```python
from build123d import *

# Parameters (mm, degrees)
SKETCH1_R           = 11.000000098
SKETCH1_R_2         = 4.1984422
SKETCH1_R_3         = 1.56235781
BOSS_EXTRUDE1_DEPTH = 2.794
SKETCH4_R           = 5.08
BOSS_EXTRUDE2_DEPTH = 5.08
BOSS_EXTRUDE4_DEPTH = 25.4


with BuildPart() as part:
    # Sketch1 → Boss-Extrude1 (new body)
    with BuildSketch(Plane.XY):
        with Locations((-211.672901702, 6.35719782)):
            Circle(SKETCH1_R)
        with Locations((-211.672901702, 6.35719782)):
            Circle(SKETCH1_R_2, mode=Mode.SUBTRACT)
        with Locations((-211.672901702, 14.35819782)):
            Circle(SKETCH1_R_3, mode=Mode.SUBTRACT)
        with Locations((-219.673901702, 6.35719782)):
            Circle(SKETCH1_R_3, mode=Mode.SUBTRACT)
        with Locations((-211.672901702, -1.64380218)):
            Circle(SKETCH1_R_3, mode=Mode.SUBTRACT)
        with Locations((-203.671901702, 6.35719782)):
            Circle(SKETCH1_R_3, mode=Mode.SUBTRACT)
    extrude(amount=BOSS_EXTRUDE1_DEPTH)

    # Sketch4 → Boss-Extrude2 (add)
    with BuildSketch(Plane.XY.offset(2.794)):
        with Locations((-211.672901702, 6.35719782)):
            Circle(SKETCH4_R)
    extrude(amount=BOSS_EXTRUDE2_DEPTH)

    # Sketch6 → Boss-Extrude4 (add)
    with BuildSketch(Plane.XY.offset(7.874)):
        Polygon((-217.614895912, 10.703116021), (-210.880223241, 13.676074856), (-204.938229031, 9.330156654), (-205.730907491, 2.011279618), (-212.465580162, -0.961679217), (-218.407574373, 3.384238985), align=None)
    extrude(amount=BOSS_EXTRUDE4_DEPTH)


solid = part.part
```
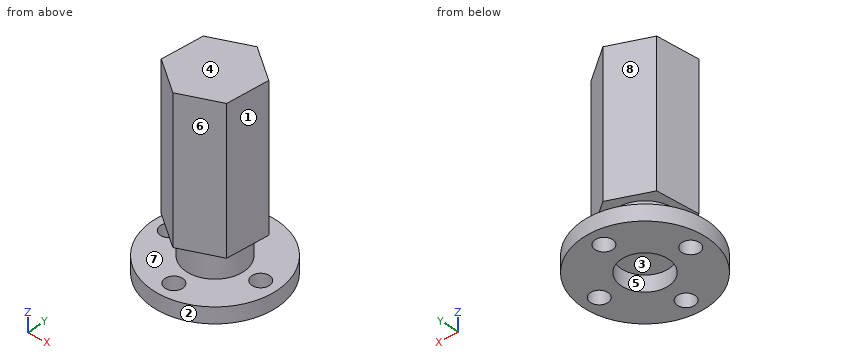
Build history of the part. All positions in model axes, mm. Face numbers are marked on the shaded views. A direction names the side the tool comes from. Give positions to 0.01 mm unless a question says otherwise; leave off trailing zeros. Order: outer loops, then holes, each group sorted by start corner. A loop starts at its lowest first (then second) coordinate and runs counter-clockwise, first axis right, second up. Notation, with made-up numbers: M 82,-9.5 L 117,-9.5 A23 cw 117,22.5 Z; hole C 45,81 d9. An arc over 180 degrees is marked long. Return JSON: item names as keys, results as strings.
Q1. Band-saw the part on D-D (z = 25). Give the cut face in (x, y), then the cut area to 3 significant figures.
Answer list:
{"outline": "M -218.41,3.38 L -212.47,-0.96 L -205.73,2.01 L -204.94,9.33 L -210.88,13.68 L -217.61,10.7 Z", "area": "141 mm^2"}
Q2. Two-plate mould, pull along X, no slides. Class the marked faces 1, 2, 3 and 4: pulls with the +X half, pulls with the -X half, needs draft (parallel to the pull), parting line crosses it, or undercut.
Answer list:
{"face 1": "pulls with the +X half", "face 2": "parting line crosses it", "face 3": "undercut", "face 4": "needs draft"}
Q3. Flat gauge pins, fed straight in: pin 1 (10 mm diameter, centred on y = -2, z = 25.5, fed in from +X); pin 2 (3 mm diameter, centred on x = -219.67, y = 6.36, fed in from +Z); pin 3 (4 mm diameter, centred on x = -211.67, y = -1.64, fed in from -Z); pin 4 (5 mm diameter, centred on x = -213, z = 18, fed in from -Y). Where does each tip first touch, or does it go through?
Answer list:
{"pin 1": "stops at x = -205.62", "pin 2": "passes through", "pin 3": "stops at z = 0", "pin 4": "stops at y = -0.96"}
Q4. 3-axis set-ups, long thin cutter, end or side, ignore diameter. For the marked faces 5, 6, 7 and 8: which of +Z, -Z, +X, -X, +Y, -Y reach the whole face in a straight line?
Answer list:
{"face 5": "-Z", "face 6": "+Z, +X, -Y", "face 7": "none", "face 8": "+Z, -X, +Y"}
Q5. Band-saw the part on C-C (y = 7). Give the cut face in (x, z), then the cut area to 3 significant figures.
Answer list:
{"outline": "M -222.65,0 L -221.1,0 L -221.1,2.79 L -222.65,2.79 Z; M -218.25,0 L -215.82,0 L -215.82,2.79 L -207.52,2.79 L -207.52,0 L -205.1,0 L -205.1,2.79 L -206.63,2.79 L -206.63,7.87 L -205.19,7.87 L -205.19,33.27 L -218.02,33.27 L -218.02,7.87 L -216.71,7.87 L -216.71,2.79 L -218.25,2.79 Z; M -202.25,0 L -200.69,0 L -200.69,2.79 L -202.25,2.79 Z", "area": "399 mm^2"}
Q6. Band-saw the part on A-A (x = -203.5). Give the cut face in (y, z), then the cut area to 3 significant figures.
Answer list:
{"outline": "M -1.01,0 L 4.8,0 L 4.8,2.79 L -1.01,2.79 Z; M 7.91,0 L 13.72,0 L 13.72,2.79 L 7.91,2.79 Z", "area": "32.5 mm^2"}
Q7. Band-saw the part on B-B (y = 15). Give the cut face in (x, z), then the cut area to 3 significant figures.
Answer list:
{"outline": "M -218.48,0 L -213.1,0 L -213.1,2.79 L -218.48,2.79 Z; M -210.25,0 L -204.87,0 L -204.87,2.79 L -210.25,2.79 Z", "area": "30.1 mm^2"}
Q8. Wall check: probe 1 along Z at (x, y) = (-215.25, 12); probe 2 along Z at (x, y) = (-213.75, 9); probe 3 along Z at (x, y) = (-208, 10.5). Give the ranges that are in metal, low to high. Write a range as from..to.
Answer list:
{"probe 1": "z = 0..2.79", "probe 2": "z = 2.79..33.27", "probe 3": "z = 0..2.79, 7.87..33.27"}
